The model under review builds one solid part; all positions refer to its coordinate system, in mm. A direction names the side the tool comes from. Coordinates: 2 decimals unless noted, no trailing zeros. Loops run counter-clockwise (first coordinate to the right, second up) from the corner with the lowest first, then second, coordinate; pieces in that order, holes last. Notation, with made-up numbers: M 76,-35.75 L 98,-35.75 A17 ccw 98,-27.75 Z; hole C 33,61 d4. An arc over 180 degrees is marked long. Return JSON: item names as keys, results as strings.
```python
from build123d import *

# Parameters (mm, degrees)
BOSS_EXTRUDE1_DEPTH     = 11
CUT_EXTRUDE1_START      = 3
SKETCH2_R               = 4.25
CUT_EXTRUDE1_DEPTH      = 4
SKETCH3_W               = 5
SKETCH3_H               = 13.464597237
CUT_EXTRUDE2_DEPTH      = 13
CUT_EXTRUDE2_DEPTH_BACK = 13
SKETCH4_W               = 7.273345506
SKETCH4_H               = 1.5
CUT_EXTRUDE3_DEPTH      = 3
SKETCH5_W               = 4.264362618
SKETCH5_H               = 2.5
CUT_EXTRUDE4_DEPTH      = 2.5
SKETCH6_W               = 5.237267166
SKETCH6_H               = 2.5
CUT_EXTRUDE5_DEPTH      = 2.5


with BuildPart() as part:
    # Sketch1 → Boss-Extrude1 (new body)
    with BuildSketch(Plane.XY):
        with BuildLine():
            Line((-11.958260743, -1), (11.958260743, -1))
            ThreePointArc((11.958260743, -1), (0, 12), (-11.958260743, -1))
        make_face()
    extrude(amount=BOSS_EXTRUDE1_DEPTH)

    # Sketch2 → Cut-Extrude1 (cut)
    with BuildSketch(Plane.XZ.offset(-2).offset(CUT_EXTRUDE1_START)):
        with Locations((0, 5.5)):
            Circle(SKETCH2_R)
    extrude(amount=-CUT_EXTRUDE1_DEPTH, mode=Mode.SUBTRACT)

    # Sketch3 → Cut-Extrude2 (cut, two sides)
    with BuildSketch(Plane(origin=(0, 0, 0), x_dir=(0, 0, -1), z_dir=(1, 0, 0))) as cut_extrude2_sk:
        with Locations((-5.5, 8.732298618)):
            Rectangle(SKETCH3_W, SKETCH3_H)
    extrude(amount=CUT_EXTRUDE2_DEPTH, mode=Mode.SUBTRACT)
    extrude(cut_extrude2_sk.sketch, amount=-CUT_EXTRUDE2_DEPTH_BACK, mode=Mode.SUBTRACT)

    # Sketch4 → Cut-Extrude3 (cut)
    with BuildSketch(Plane.XY.offset(11)):
        with Locations((10.094933496, -0.25)):
            Rectangle(SKETCH4_W, SKETCH4_H)
    extrude(amount=-CUT_EXTRUDE3_DEPTH, mode=Mode.SUBTRACT)

    # Sketch5 → Cut-Extrude4 (cut)
    with BuildSketch(Plane.XY.offset(11)):
        with Locations((-10.590442052, 0.25)):
            Rectangle(SKETCH5_W, SKETCH5_H)
    extrude(amount=-CUT_EXTRUDE4_DEPTH, mode=Mode.SUBTRACT)

    # Sketch6 → Cut-Extrude5 (cut)
    with BuildSketch(Plane.XY.offset(11)):
        with Locations((11.076894326, 0.25)):
            Rectangle(SKETCH6_W, SKETCH6_H)
    extrude(amount=-CUT_EXTRUDE5_DEPTH, mode=Mode.SUBTRACT)


solid = part.part
```
1. Add section C-C on x = 0. Give the boundary of the cut face in (y, z).
Check values:
{"outline": "M -1,0 L 12,0 L 12,3 L 3,3 L 3,1.25 L -1,1.25 Z; M -1,9.75 L 3,9.75 L 3,8 L 12,8 L 12,11 L -1,11 Z"}
2. Add section B-B on z = 5.5. Give the boundary of the cut face in (x, y), plus the area to 3 significant figures.
Check values:
{"outline": "M -11.96,-1 L -4.25,-1 L -4.25,2 L -11.83,2 A12 ccw Z; M 4.25,-1 L 11.96,-1 A12 ccw 11.83,2 L 4.25,2 Z", "area": "46.2 mm²"}
3. To check wall thickness, follow line 1 (Z direction, x = 0, y = 1.1); line 2 (Z direction, x = 2, y = 6); line 3 (Y direction, x = 8.5, z = 6.75). State the ranges of each line that lie inside material, in increasing order.
Check values:
{"line 1": "0 to 1.25, 9.75 to 11", "line 2": "0 to 3, 8 to 11", "line 3": "-1 to 2"}
4. Machinability: for faces 1 (the face through (-4.246, 0.972, 5.687)), 2 (the face through (0, 6, 8)), 3 (the face through (-8.458, 0, 10)), which of the approach directions +Z, -Z, +X, -X, +Y, -Y give a long, thin tool a straight path to every point of the face, cutting with its end or side? Answer none if there is none.
Check values:
{"face 1": "-Y", "face 2": "+X, -X, +Y", "face 3": "+Z, -X, -Y"}
5. Add section D-D on y = 4. Give the boundary of the cut face in (x, z), plus the area to 3 significant figures.
Check values:
{"outline": "M -11.31,0 L 11.31,0 L 11.31,3 L -11.31,3 Z; M -11.31,8 L 11.31,8 L 11.31,11 L -11.31,11 Z", "area": "136 mm²"}
6. Add section A-A on y = 0. Give the boundary of the cut face in (x, z).
Check values:
{"outline": "M -12,0 L 12,0 L 12,8 L 6.46,8 L 6.46,11 L -8.46,11 L -8.46,8.5 L -12,8.5 Z; hole C 0,5.5 d8.5"}
7. Insertion check: pin 1 Ø1.9 at (x, z) = (-0.5, 8.5) entering from -Y; pin 2 Ø0.8 at (y, z) = (-0.5, 9) entering from +X; pin 3 Ø1.5 at (y, z) = (8, 3) entering from +X. Each pin has a flat end and moves straight along its axis. Give the tip position at first contact, or say it passes through.
Check values:
{"pin 1": "y = 3", "pin 2": "x = 6.46", "pin 3": "x = 9.56"}
8. The part is to be moulded in two halves that separate along Z. For faces 4 (the face through (10, 1, 8.5)), 5 (the face through (8, 2, 6)), 6 (the face through (-3, -1, 2)), say which applies: released by +Z, released by -Z, zero draft, split by the parting line, or undercut.
Check values:
{"face 4": "released by +Z", "face 5": "undercut", "face 6": "zero draft"}
